Geometry check sheet. Reference: the model listing, model coordinates, mm. Face numbers are marked on the shaded views. Coordinates: 2 decimals unless noted, no trailing zeros. Order: outer loops, then holes, each group sorted by start corner. A loop starts at its lowest first (then second) coordinate and runs counter-clockwise, first axis right, second up. Notation, with made-up numbers: (78.5, 13) - (124.5, 13) arc R13 ccw to (124.5, 31) - close; hole circle Ø7 at (-23, -30). An arc over 180 degrees is marked (long way). Return JSON: item names as keys, results as strings. Group by question number.
Item 1: Section check D-D on y = 4.25. Enter the section's corners in (x, z).
Item 2: Gauge pin test, flat ends, axial feed: pin 1 (2 mm diameter, centred on y = 3, z = -11, fed in from -X); pin 2 (2 mm diameter, centred on x = 0, y = 0, fed in from +Z); pin 3 (6 mm diameter, centred on x = 3.5, z = -17, fed in from -Y). Record the tip position at first contact, or that the pin passes through.
Item 3: Draft check along X on the marked faces 1, 2 and 3. Enter one of: pulls with the +X half, pulls with the -X half, needs draft (parallel to the pull), parting line crosses it, or undercut.
Item 4: Section check C-C on x = -4. Enter the section's corners in (y, z).
Item 5: Section check A-A on y = 0. Enter the section's corners in (x, z) (1 decimal).
Item 6: Scan lines: probe 1 along X at (y, z) = (1, -1.75); probe 2 along Z at (x, y) = (-1, -1.5); probe 3 along X at (y, z) = (2.5, -18). Record each from-to range of solid material in increasing order.
Item 7: Section check B-B on z = -9. Enter the section's corners in (x, y) (3 decimals).
from build123d import *

# Parameters (mm, degrees)
SKETCH1_W          = 19.05
SKETCH1_H          = 3.175
CHAMFER1_SIZE      = 0.9525
CUT_EXTRUDE2_DEPTH = 2.34696


with BuildPart() as part:
    # Sketch1 → Revolve1 (revolve)
    with BuildSketch(Plane(origin=(0, 0, 0), x_dir=(0, 0, -1), z_dir=(1, 0, 0))):
        with Locations((12.8778, 1.5875)):
            Rectangle(SKETCH1_W, SKETCH1_H)
    revolve(axis=Axis((0, 0, -22.4028), (0, 0, 1)))

    # Chamfer1
    chamfer1_edges = [part.edges().sort_by_distance(p)[0] for p in [
        (0, -3.175, -22.4028),
    ]]
    chamfer(chamfer1_edges, length=CHAMFER1_SIZE)

    # Sketch7 → Revolve2 (revolve)
    with BuildSketch(Plane(origin=(0, 0, 0), x_dir=(0, 0, -1), z_dir=(1, 0, 0)), mode=Mode.PRIVATE) as revolve2_sk:
        with BuildLine():
            Line((2.84988, 5.5499), (3.3528, 5.5499))
            Line((3.3528, 5.5499), (3.3528, 0))
            Line((3.3528, 0), (0, 0))
            Line((0, 0), (0, 3.175))
            ThreePointArc((0, 3.175), (1.235921075, 4.58927271), (2.84988, 5.5499))
        make_face()
    revolve(revolve2_sk.sketch.rotate(Axis((0, 0, 0), (0, 0, -1)), 180), axis=Axis((0, 0, 0), (0, 0, -1)))

    # Sketch5 → Cut-Extrude2 (cut)
    with BuildSketch(Plane.XY):
        Polygon((1.984375, -1.14567944), (1.984375, 1.14567944), (0, 2.291358881), (-1.984375, 1.14567944), (-1.984375, -1.14567944), (0, -2.291358881), align=None)
    extrude(amount=-CUT_EXTRUDE2_DEPTH, mode=Mode.SUBTRACT)

    # Cut-Extrude3 cone 1 section (on through the dimple's axis) → Cut-Extrude3 (revolve, cut)
    with BuildSketch(Plane(origin=(0, 0, 0), x_dir=(0, -1, 0), z_dir=(1, 0, 0))):
        Polygon((0, 0), (2.291358881, 0), (0, 2.291358881), align=None)
    revolve(axis=Axis((0, 0, 0), (0, 0, -1)), mode=Mode.SUBTRACT)


solid = part.part
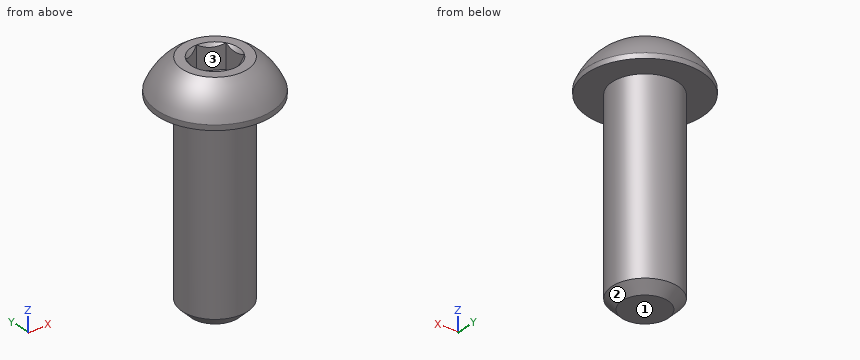
Computed:
{
 "1": {"outline": "(-3.57, -3.35) - (3.57, -3.35) - (3.57, -2.85) arc R4.2 ccw to (-3.57, -2.85) - close"},
 "2": {"pin 1": "stops at x = -2.47", "pin 2": "stops at z = -2.35", "pin 3": "stops at y = -3.14"},
 "3": {"face 1": "needs draft", "face 2": "parting line crosses it", "face 3": "undercut"},
 "4": {"outline": "(-3.85, -3.35) - (3.85, -3.35) - (3.85, -2.85) arc R4.44 ccw to (-3.85, -2.85) - close"},
 "5": {"outline": "(-5.5, -3.4) - (-3.2, -3.4) - (-3.2, -21.5) - (-2.2, -22.4) - (2.2, -22.4) - (3.2, -21.5) - (3.2, -3.4) - (5.5, -3.4) - (5.5, -2.8) arc R6 ccw to (3.2, 0) - (2.3, 0) - (2, -0.3) - (2, -2.3) - (-2, -2.3) - (-2, -0.3) - (-2.3, 0) - (-3.2, 0) arc R6 ccw to (-5.5, -2.8) - close"},
 "6": {"probe 1": "x = -4.87 to -1.98, 1.98 to 4.87", "probe 2": "z = -22.4 to -2.35", "probe 3": "x = -1.96 to 1.96"},
 "7": {"outline": "circle Ø6.35 at (0, 0)"}
}
